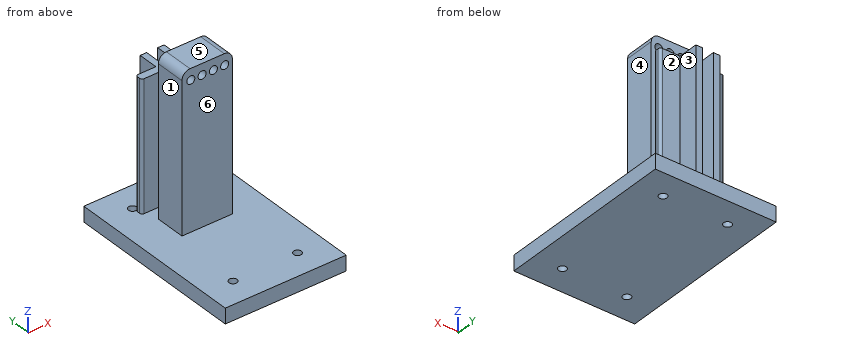
```python
from build123d import *

# Parameters (mm, degrees)
SKETCH1_W            = 38.1
SKETCH1_H            = 57.15
BOSS_EXTRUDE1_DEPTH  = 4.7625
SKETCH2_R            = 1.2446
CUT_EXTRUDE1_DEPTH   = 4.7625
SKETCH4_W            = 15.875
SKETCH4_H            = 9.525
BOSS_EXTRUDE2_DEPTH  = 49.2125
CUT_EXTRUDE2_REACH   = 72.568
SKETCH5_R            = 1.27
FILLET2_R            = 2.54
SKETCH8_W            = 2.032
SKETCH8_H            = 12.684715198
BOSS_EXTRUDE4_DEPTH  = 40.64
SKETCH9_W            = 40.552264906
SKETCH9_H            = 2.38125
BOSS_EXTRUDE5_DEPTH  = 6.35
FILLET4_R            = 0.762
FILLET4_OF_MIRROR2_R = 0.762


with BuildPart() as part:
    # Sketch1 → Boss-Extrude1 (new body)
    with BuildSketch(Plane.XY):
        Rectangle(SKETCH1_W, SKETCH1_H)
    extrude(amount=BOSS_EXTRUDE1_DEPTH)

    # Sketch2 → Cut-Extrude1 (cut)
    with BuildSketch(Plane.XY):
        with Locations(Location((10.16, 20.32, 0), (0, 0, 180))):
            Circle(SKETCH2_R)
        with Locations(Location((-10.16, 20.32, 0), (0, 0, 180))):
            Circle(SKETCH2_R)
        with Locations(Location((10.16, -20.32, 0), (0, 0, 180))):
            Circle(SKETCH2_R)
        with Locations(Location((-10.16, -20.32, 0), (0, 0, 180))):
            Circle(SKETCH2_R)
    extrude(amount=CUT_EXTRUDE1_DEPTH, mode=Mode.SUBTRACT)

    # Sketch4 → Boss-Extrude2 (add)
    with BuildSketch(Plane.XY.offset(4.7625)):
        with Locations((0, 7.9375)):
            Rectangle(SKETCH4_W, SKETCH4_H)
    extrude(amount=BOSS_EXTRUDE2_DEPTH)

    # Sketch5 → Cut-Extrude2 (cut, up to next)
    with BuildSketch(Plane(origin=(0, 12.7, 0), x_dir=(1, 0, 0), z_dir=(0, 1, 0)), mode=Mode.PRIVATE) as cut_extrude2_sk1:
        with Locations(Location((-5.1435, -50.4825, 0), (0, 0, 180))):
            Circle(SKETCH5_R)
    cut_extrude2_tool1 = extrude(cut_extrude2_sk1.sketch, amount=-CUT_EXTRUDE2_REACH, mode=Mode.PRIVATE) & part.part
    # Sketch5 → Cut-Extrude2 (cut, up to next)
    with BuildSketch(Plane(origin=(0, 12.7, 0), x_dir=(1, 0, 0), z_dir=(0, 1, 0)), mode=Mode.PRIVATE) as cut_extrude2_sk2:
        with Locations(Location((-1.5875, -50.4825, 0), (0, 0, 180))):
            Circle(SKETCH5_R)
    cut_extrude2_tool2 = extrude(cut_extrude2_sk2.sketch, amount=-CUT_EXTRUDE2_REACH, mode=Mode.PRIVATE) & part.part
    # Sketch5 → Cut-Extrude2 (cut, up to next)
    with BuildSketch(Plane(origin=(0, 12.7, 0), x_dir=(1, 0, 0), z_dir=(0, 1, 0)), mode=Mode.PRIVATE) as cut_extrude2_sk3:
        with Locations(Location((1.9685, -50.4825, 0), (0, 0, 180))):
            Circle(SKETCH5_R)
    cut_extrude2_tool3 = extrude(cut_extrude2_sk3.sketch, amount=-CUT_EXTRUDE2_REACH, mode=Mode.PRIVATE) & part.part
    # Sketch5 → Cut-Extrude2 (cut, up to next)
    with BuildSketch(Plane(origin=(0, 12.7, 0), x_dir=(1, 0, 0), z_dir=(0, 1, 0)), mode=Mode.PRIVATE) as cut_extrude2_sk4:
        with Locations(Location((5.5245, -50.4825, 0), (0, 0, 180))):
            Circle(SKETCH5_R)
    cut_extrude2_tool4 = extrude(cut_extrude2_sk4.sketch, amount=-CUT_EXTRUDE2_REACH, mode=Mode.PRIVATE) & part.part
    add(cut_extrude2_tool1.solids().sort_by_distance((-5.1435, 12.7, 50.4825))[0], mode=Mode.SUBTRACT)
    add(cut_extrude2_tool2.solids().sort_by_distance((-1.5875, 12.7, 50.4825))[0], mode=Mode.SUBTRACT)
    add(cut_extrude2_tool3.solids().sort_by_distance((1.9685, 12.7, 50.4825))[0], mode=Mode.SUBTRACT)
    add(cut_extrude2_tool4.solids().sort_by_distance((5.5245, 12.7, 50.4825))[0], mode=Mode.SUBTRACT)

    # Fillet2
    fillet2_edges = [part.edges().sort_by_distance(p)[0] for p in [
        (-7.9375, 7.9375, 53.975),
        (7.9375, 7.9375, 53.975),
    ]]
    fillet(fillet2_edges, radius=FILLET2_R)

    # Sketch8 → Boss-Extrude4 (add)
    with BuildSketch(Plane.XY.offset(4.7625)):
        with Locations((-2.76225, 19.042357599)):
            Rectangle(SKETCH8_W, SKETCH8_H)
        with Locations((2.76225, 19.042357599)):
            Rectangle(SKETCH8_W, SKETCH8_H)
    extrude(amount=BOSS_EXTRUDE4_DEPTH)

    # Sketch9 → Boss-Extrude5 (add)
    with BuildSketch(Plane.ZY.offset(3.77825)):
        with Locations((25.126367547, 17.859375)):
            Rectangle(SKETCH9_W, SKETCH9_H)
    boss_extrude5 = extrude(amount=BOSS_EXTRUDE5_DEPTH)

    # Fillet4
    fillet4_edges = [part.edges().sort_by_distance(p)[0] for p in [
        (-10.12825, 19.05, 25.126367547),
        (-10.12825, 16.66875, 25.126367547),
    ]]
    fillet(fillet4_edges, radius=FILLET4_R)

    # Mirror2: Boss-Extrude5 across plane
    add(boss_extrude5.mirror(Plane.ZY))

    # Fillet4 of Mirror2
    fillet4_of_mirror2_edges = [part.edges().sort_by_distance(p)[0] for p in [
        (10.12825, 19.05, 25.126367547),
        (10.12825, 16.66875, 25.126367547),
    ]]
    fillet(fillet4_of_mirror2_edges, radius=FILLET4_OF_MIRROR2_R)


solid = part.part
```
Work out the finished part from the listing and answer in its coordinate system (mm). Face numbers are marked on the shaded views. A direction names the side the tool comes from. Coordinates: 2 decimals unless noted, no trailing zeros. Loops run counter-clockwise (first coordinate to the right, second up) from the corner with the lowest first, then second, coordinate; pieces in that order, holes last.
1) Flat-ended cylindrical pins translate along their axes: pin 1 (3 mm diameter, centred on x = 8, z = 19.5, fed in from -Y) (3 decimals); pin 2 (12.5 mm diameter, centred on x = 1, z = 28.5, fed in from +Y); pin 3 (6.5 mm diameter, centred on y = 19, z = 16, fed in from -X); pin 4 (2 mm diameter, centred on x = -1.59, z = 50.48, fed in from +Y). Find the tip coordinate at first contact, or state that the pin passes through.
Results:
pin 1: stops at y = 3.175
pin 2: stops at y = 25.38
pin 3: stops at x = -10.13
pin 4: passes through
2) For a pull along Y with two mould halves and no side action, classify the marked faces 1, 2 and 3 as +Y half, -Y half, draft (parallel to the pull), parting line (faces both ways), or undercut.
Results:
face 1: draft
face 2: +Y half
face 3: undercut
3) Section C-C (y = 20.32) is taken. Give the vertices of the cut face in (x, z).
Results:
outline: (-19.05, 0) - (-11.4, 0) - (-11.4, 4.76) - (-19.05, 4.76) - close; (-8.92, 0) - (8.92, 0) - (8.92, 4.76) - (3.78, 4.76) - (3.78, 45.4) - (1.75, 45.4) - (1.75, 4.76) - (-1.75, 4.76) - (-1.75, 45.4) - (-3.78, 45.4) - (-3.78, 4.76) - (-8.92, 4.76) - close; (11.4, 0) - (19.05, 0) - (19.05, 4.76) - (11.4, 4.76) - close
4) For the marked faces 4, 5 and 6, determine the directions among +Z, -Z, +X, -X, +Y, -Y from which every point of the face is accessible in a straight line to the end or side of a thin tool.
Results:
face 4: +Z, +X, -Y
face 5: +Z, +X, -X, +Y, -Y
face 6: +Z, +X, -X, -Y
5) Consider probe 1 along Y at (x, z) = (10.16, 3.25) (3 decimals); probe 2 along X at (y, z) = (23, 18); probe 3 along Y at (x, z) = (4.5, 34) (3 decimals). Determine where each line is inside the solid, lowest interval first.
Results:
probe 1: y = -28.575 to -21.565, -19.075 to 19.075, 21.565 to 28.575
probe 2: x = -3.78 to -1.75, 1.75 to 3.78
probe 3: y = 3.175 to 12.7, 16.669 to 19.05
6) Section D-D (y = 14) is taken. Give the vertices of the cut face in (x, z).
Results:
outline: (-19.05, 0) - (19.05, 0) - (19.05, 4.76) - (3.78, 4.76) - (3.78, 45.4) - (1.75, 45.4) - (1.75, 4.76) - (-1.75, 4.76) - (-1.75, 45.4) - (-3.78, 45.4) - (-3.78, 4.76) - (-19.05, 4.76) - close
7) Section A-A (y = -20.32) is taken. Give the vertices of the cut face in (x, z).
Results:
outline: (-19.05, 0) - (-11.4, 0) - (-11.4, 4.76) - (-19.05, 4.76) - close; (-8.92, 0) - (8.92, 0) - (8.92, 4.76) - (-8.92, 4.76) - close; (11.4, 0) - (19.05, 0) - (19.05, 4.76) - (11.4, 4.76) - close
